The model under review builds one solid part; all positions refer to its coordinate system, in mm. Face numbers are marked on the shaded views. A direction names the side the tool comes from. Coordinates: 2 decimals unless noted, no trailing zeros. Order: outer loops, then holes, each group sorted by start corner. A loop starts at its lowest first (then second) coordinate and runs counter-clockwise, first axis right, second up.
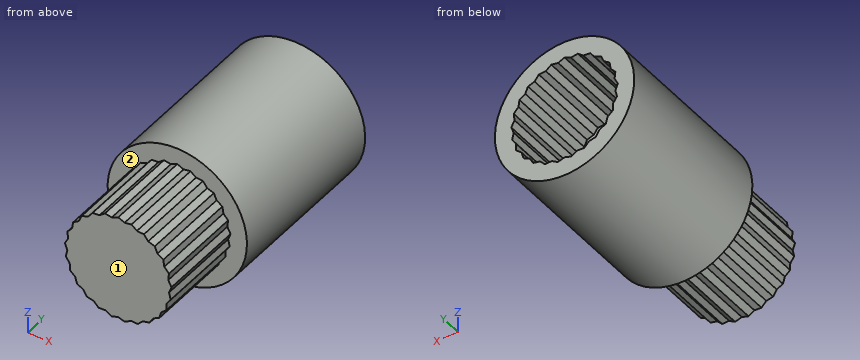
```python
from build123d import *

# Parameters (mm, degrees)
BOSS_EXTRUDE2_DEPTH = 5
SKETCH2_R           = 4
BOSS_EXTRUDE3_DEPTH = 10
CUT_EXTRUDE4_DEPTH  = 5


with BuildPart() as part:
    # Sketch1 → Boss-Extrude2 (new body)
    with BuildSketch(Plane(origin=(0, 0, 0), x_dir=(1, 0, 0), z_dir=(0, 1, 0))):
        Polygon((0, 2.925), (-0.384146361, 3.04083156), (-0.72741792, 2.833105746), (-1.128301754, 2.849764929), (-1.409129497, 2.563197039), (-1.801561798, 2.479637088), (-2.002300285, 2.132233235), (-2.361623089, 1.953704529), (-2.469659182, 1.567293375), (-2.773294916, 1.305013529), (-2.78184031, 0.903874709), (-3.010710423, 0.574323729), (-2.919228181, 0.18366227), (-3.058951923, -0.192452942), (-2.873190208, -0.548090345), (-2.914988222, -0.947137088), (-2.646619128, -1.245404428), (-2.587865092, -1.642309127), (-2.253751235, -1.86446517), (-2.09813688, -2.234288843), (-1.719271863, -2.366374709), (-1.476575011, -2.685879974), (-1.076764317, -2.719596221), (-0.762234504, -2.968707389), (-0.366599708, -2.901935501), (0, -3.065), (0.366599708, -2.901935501), (0.762234504, -2.968707389), (1.076764317, -2.719596221), (1.476575011, -2.685879974), (1.719271863, -2.366374709), (2.09813688, -2.234288843), (2.253751235, -1.86446517), (2.587865092, -1.642309127), (2.646619128, -1.245404428), (2.914988222, -0.947137088), (2.873190208, -0.548090345), (3.058951923, -0.192452942), (2.919228181, 0.18366227), (3.010710423, 0.574323729), (2.78184031, 0.903874709), (2.773294916, 1.305013529), (2.469659182, 1.567293375), (2.361623089, 1.953704529), (2.002300285, 2.132233235), (1.801561798, 2.479637088), (1.409129497, 2.563197039), (1.128301754, 2.849764929), (0.72741792, 2.833105746), (0.384146361, 3.04083156), align=None)
    extrude(amount=BOSS_EXTRUDE2_DEPTH)

    # Sketch2 → Boss-Extrude3 (add)
    with BuildSketch(Plane(origin=(0, 5, 0), x_dir=(1, 0, 0), z_dir=(0, 1, 0))):
        with Locations(Location((0, 0, 0), (0, 0, 270))):
            Circle(SKETCH2_R)
    extrude(amount=BOSS_EXTRUDE3_DEPTH)

    # Sketch3 → Cut-Extrude4 (cut)
    with BuildSketch(Plane(origin=(0, 15, 0), x_dir=(1, 0, 0), z_dir=(0, 1, 0))):
        Polygon((-0.72741792, 2.833105746), (-0.384146361, 3.04083156), (0, 2.925), (0.384146361, 3.04083156), (0.72741792, 2.833105746), (1.128301754, 2.849764929), (1.409129497, 2.563197039), (1.801561798, 2.479637088), (2.002300285, 2.132233235), (2.361623089, 1.953704529), (2.469659182, 1.567293375), (2.773294916, 1.305013529), (2.78184031, 0.903874709), (3.010710423, 0.574323729), (2.919228181, 0.18366227), (3.058951923, -0.192452942), (2.873190208, -0.548090345), (2.914988222, -0.947137088), (2.646619128, -1.245404428), (2.587865092, -1.642309127), (2.253751235, -1.86446517), (2.09813688, -2.234288843), (1.719271863, -2.366374709), (1.476575011, -2.685879974), (1.076764317, -2.719596221), (0.762234504, -2.968707389), (0.366599708, -2.901935501), (0, -3.065), (-0.366599708, -2.901935501), (-0.762234504, -2.968707389), (-1.076764317, -2.719596221), (-1.476575011, -2.685879974), (-1.719271863, -2.366374709), (-2.09813688, -2.234288843), (-2.253751235, -1.86446517), (-2.587865092, -1.642309127), (-2.646619128, -1.245404428), (-2.914988222, -0.947137088), (-2.873190208, -0.548090345), (-3.058951923, -0.192452942), (-2.919228181, 0.18366227), (-3.010710423, 0.574323729), (-2.78184031, 0.903874709), (-2.773294916, 1.305013529), (-2.469659182, 1.567293375), (-2.361623089, 1.953704529), (-2.002300285, 2.132233235), (-1.801561798, 2.479637088), (-1.409129497, 2.563197039), (-1.128301754, 2.849764929), align=None)
    extrude(amount=-CUT_EXTRUDE4_DEPTH, mode=Mode.SUBTRACT)


solid = part.part
```
(1) We need section C-C, the plane x = 3.25. Write out the cut boundary in (y, z).
A:
outline: (5, -2.33) - (15, -2.33) - (15, 2.33) - (5, 2.33) - close
(2) For pin 1 Ø2 at (y, z) = (6.5, 1.5) entering from -X; pin 2 Ø1.5 at (x, y) = (3, 12.5) entering from +Z; pin 3 Ø1 at (x, y) = (1, 5) entering from -Z, all flat-tipped, find the tip position at first contact; note any pin that passes through.
A:
pin 1: stops at x = -3.97
pin 2: stops at z = 3.31
pin 3: stops at z = -3.97
(3) Wall thickness on probe 1 along Y at (x, z) = (-1.5, 0.75); probe 2 along X at (y, z) = (12.75, -1.5); probe 3 along X at (y, z) = (11.25, -2): over which ranges is each line inside the solid? List them lowest first.
A:
probe 1: y = 0 to 10
probe 2: x = -3.71 to -2.55, 2.55 to 3.71
probe 3: x = -3.46 to -2.27, 2.27 to 3.46
(4) We need section A-A, the plane z = 0. Write out the cut boundary in (x, y).
A:
outline: (-4, 5) - (-2.99, 5) - (-2.99, 0) - (2.99, 0) - (2.99, 5) - (4, 5) - (4, 15) - (2.99, 15) - (2.99, 10) - (-2.99, 10) - (-2.99, 15) - (-4, 15) - close
(5) We need section D-D, the plane z = -3.25. Write out the cut boundary in (x, y), and give its area (3 significant figures).
A:
outline: (-2.33, 5) - (2.33, 5) - (2.33, 15) - (-2.33, 15) - close
area: 46.6 mm2
(6) We need section B-B, the plane y = 9.75. Write out the cut boundary in (x, z), and give its area (3 significant figures).
A:
outline: circle Ø8 at (0, 0)
area: 50.3 mm2
(7) Machinability: for the marked faces 1 and 2, which of the approach directions +Z, -Z, +X, -X, +Y, -Y give a long, thin tool a straight path to every point of the face, cutting with its end or side? Answer none if there is none.
A:
face 1: +Z, -Z, +X, -X, -Y
face 2: -Y
